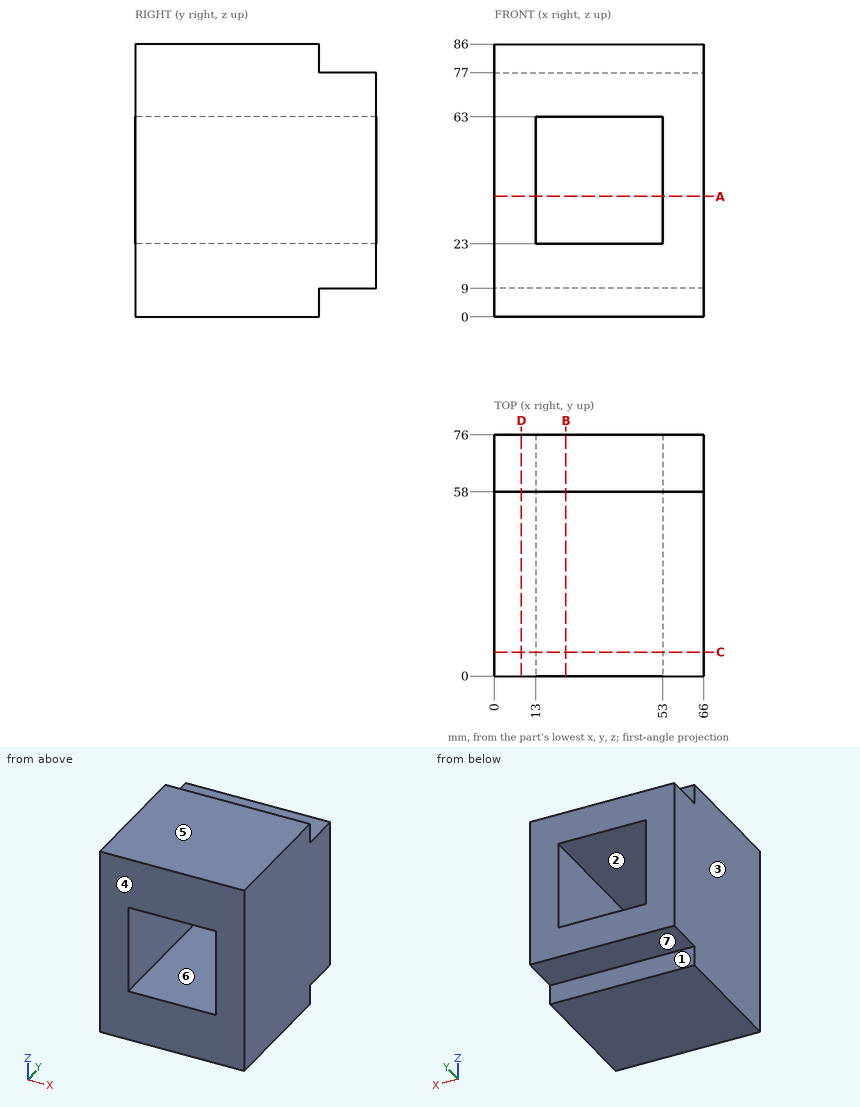
Input: dimensioned drawing with shaded views. Units: mm. Origin: part minimum x, y, z. A direction names the side the tool comes from. Give positions to 0.01 mm unless a question says otherwise; leave off trailing zeros. Write each loop counter-clockwise with the first axis right and the second up, starting at its lowest first coordinate (ties: lowest second). Pieces come first, ordered by that corner, then holes.
Q1. Section B-B, the plane x = 22.5. Output: boundary loops of the cut face in (y, z), plus the area to 3 significant figures.
Q2. Material intervals for probe 1 along X at (y, z) = (6.5, 54); probe 2 along Z at (x, y) = (14.5, 71); probe 3 along Z at (x, y) = (27.5, 46.5), sorted ascending.
Q3. Section C-C, the plane y = 7.5. Output: boundary loops of the cut face in (x, z).
Q4. First-contact query: P1, Ø5.5, axis at x = 20.5, y = 68, coming from the +Z side; P2, Ø10, axis at x = 30.5, z = 3, coming from the +Y side. Flat tips, straight axial feed; report the tip coordinate or a pass-through.
Q5. Section D-D, the plane x = 8.5. Output: boundary loops of the cut face in (y, z), plus the area to 3 significant figures.
Q6. Section A-A, the plane z = 38. Output: boundary loops of the cut face in (x, y), plus the area to 3 significant figures.
Q7. Pull-direction query (Z, two-part tool) for the marked faces 4, 5, 6 and 7; classes: pulls with the +Z half, pulls with the -Z half, needs draft (parallel to the pull), parting line crosses it, or undercut.
Q8. Set-up query: the marked faces 1, 2 and 3. Return all of +Z, -Z, +X, -X, +Y, -Y with unobstructed straight access to the full face (end or side cutting, diameter ignored); none if empty.
Filled in:
1. outline: (0, 0) - (58, 0) - (58, 9) - (76, 9) - (76, 23) - (0, 23) - close; (0, 63) - (76, 63) - (76, 77) - (58, 77) - (58, 86) - (0, 86) - close
1. area: 3,170 mm2
2. probe 1: x = 0 to 13, 53 to 66
2. probe 2: z = 9 to 23, 63 to 77
2. probe 3: z = 0 to 23, 63 to 86
3. outline: (0, 0) - (66, 0) - (66, 86) - (0, 86) - close; hole (13, 23) - (53, 23) - (53, 63) - (13, 63) - close
4. P1: stops at z = 77
4. P2: stops at y = 58
5. outline: (0, 0) - (58, 0) - (58, 9) - (76, 9) - (76, 77) - (58, 77) - (58, 86) - (0, 86) - close
5. area: 6,210 mm2
6. outline: (0, 0) - (13, 0) - (13, 76) - (0, 76) - close; (53, 0) - (66, 0) - (66, 76) - (53, 76) - close
6. area: 1,980 mm2
7. face 4: needs draft
7. face 5: pulls with the +Z half
7. face 6: undercut
7. face 7: pulls with the -Z half
8. face 1: -Z, +X, -X, +Y
8. face 2: +Y, -Y
8. face 3: +Z, -Z, -X, +Y, -Y
